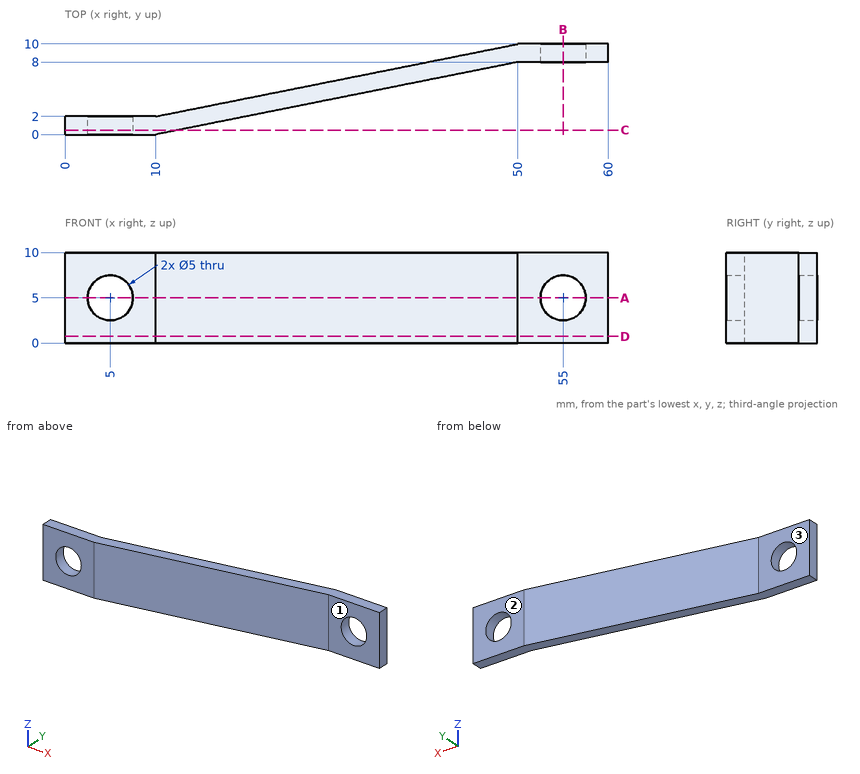
Print and shaded views of the part. All mm, measured from the part's lowest x, y and z. A direction names the side the tool comes from. Coordinates: 2 decimals unless noted, no trailing zeros. Order: outer loops, then holes, each group sorted by start corner. A loop starts at its lowest first (then second) coordinate and runs counter-clockwise, first axis right, second up. Notation, with made-up numbers: M -24.75,60 L -0.75,60 A13 cw -0.75,79 Z; hole C 22,-19.5 d6. An arc over 180 degrees is marked long. Answer as CSV lines item,"result".
1) Flat gauge pins, fed straight in: P1, Ø6, axis at x = 41.5, z = 5, coming from the +Y side; P2, Ø3, axis at x = 56, z = 5.5, coming from the -Y side; P3, Ø5, axis at x = 3, z = 5.5, coming from the +Y side. Where does each tip first touch, or does it go through?
Verdict:
P1,"y = 8.9"
P2,"y = 8"
P3,"y = 2"
2) 3-axis set-ups, long thin cutter, end or side, ignore diameter. For the marked faces 1, 2 and 3: which of +Z, -Z, +X, -X, +Y, -Y reach the whole face in a straight line?
Verdict:
face 1,"+Z, -Z, +X, -Y"
face 2,"+Z, -Z, +X, -X, +Y"
face 3,"+Z, -Z, -X, +Y"
3) Cut at B-B (x = 55). List the corners of the cut face in (y, z).
Verdict:
outline,"M 8,0 L 10,0 L 10,2.5 L 8,2.5 Z; M 8,7.5 L 10,7.5 L 10,10 L 8,10 Z"
4) Cut at C-C (y = 0.5). List the corners of the cut face in (x, z), then the cut area to 3 significant figures.
Verdict:
outline,"M 0,0 L 12.5,0 L 12.5,10 L 0,10 Z; hole C 5,5 d5"
area,"105 mm2"
5) Cut at D-D (z = 0.75). List the corners of the cut face in (x, y).
Verdict:
outline,"M 0,0 L 10,0 L 50,8 L 60,8 L 60,10 L 50,10 L 10,2 L 0,2 Z"
6) Cut at A-A (z = 5). List the corners of the cut face in (x, y), then the cut area to 4 significant figures.
Verdict:
outline,"M 0,0 L 2.5,0 L 2.5,2 L 0,2 Z; M 7.5,0 L 10,0 L 50,8 L 52.5,8 L 52.5,10 L 50,10 L 10,2 L 7.5,2 Z; M 57.5,8 L 60,8 L 60,10 L 57.5,10 Z"
area,"100.0 mm2"
7) Drill centre lines: L1, parallel to Z at x = 55, y = 9.1; L2, parallel to Y at x = 9.5, z = 2.75; L3, parallel to Y at x = 43, z = 8.25. Where is each one in solid material? Low to high. Write a range as from..to.
Verdict:
L1,"0..2.5, 7.5..10"
L2,"0..2"
L3,"6.6..8.6"
